Autodesk Inventor part; units mm, degrees
ref_plane "YZ Plane" through (0, 0, 0) normal (1, 0, 0) x (0, 1, 0)
ref_plane "XZ Plane" through (0, 0, 0) normal (0, 1, 0) x (-1, 0, 0)
ref_plane "XY Plane" through (0, 0, 0) normal (0, 0, 1) x (1, 0, 0)
sketch "Sketch1" plane through (0, 0, 0) normal (0, 1, 0) x (-1, 0, 0)
  line L0 (8, 8) -> (-8, 8) construction
  line L1 (-8, 8) -> (-8, -8) construction
  line L2 (-8, -8) -> (8, -8) construction
  line L3 (8, -8) -> (8, 8) construction
  line L4 (8, 8) -> (-8, -8) construction
  line L5 (-8, 8) -> (8, -8) construction
  line L6 (-8.25, 8.25) -> (8.25, 8.25)
  line L7 (8.25, 8.25) -> (8.25, -8.25)
  line L8 (8.25, -8.25) -> (-8.25, -8.25)
  line L9 (-8.25, -8.25) -> (-8.25, 8.25)
  line L10 (-8.25, 8.25) -> (8.25, -8.25) construction
  line L11 (8.25, 8.25) -> (-8.25, -8.25) construction
  line L12 (-10.25, 10.25) -> (10.25, 10.25)
  line L13 (10.25, 10.25) -> (10.25, -10.25)
  line L14 (10.25, -10.25) -> (-10.25, -10.25)
  line L15 (-10.25, -10.25) -> (-10.25, 10.25)
  line L16 (-10.25, 10.25) -> (10.25, -10.25) construction
  line L17 (10.25, 10.25) -> (-10.25, -10.25) construction
  circle A0 centre (2.8, -4.25) radius 1.75
  circle A1 centre (-2.8, -4.25) radius 1.75
  line L18 (7.25, -7.25) -> (-7.25, -7.25)
  line L19 (-7.25, -1.25) -> (7.25, -1.25)
  line L20 (7.25, -1.25) -> (7.25, -7.25)
  line L21 (-7.25, -1.25) -> (-7.25, -7.25)
  line L22 (-6.75, 8.25) -> (-6.75, 10.25)
  line L23 (0, 8.25) -> (0, 10.25)
  point P0 (0, 0)
  point P1 (0, -1.25)
  point P2 (7.25, -4.25)
  dimension "d0" = 16
  dimension "d1" = 16.5
  dimension "d2" = 2
  dimension "d3" = 3.5
  dimension "d4" = 5.6
  dimension "d5" = 2.8
  dimension "d6" = 6
  dimension "d7" = 1
  dimension "d8" = 1
  dimension "d15" = 1.5
extrude "Extrusion1" add sketch "Sketch1" along normal blind 1.5 contours L9 L8 L7 L6 L23 L12 L13 L14 L15 L22
extrude "Extrusion2" add sketch "Sketch1" against normal blind 1.5 contours L9 L8 L7 L6 L23 L12 L13 L14 L15 L22 | L6 L7 L8 L9 | L22 L12 L23 L6
sketch "Sketch2" plane through (0, -1.5, 0) normal (0, -1, 0) x (1, 0, 0)
  line L0 (-10.25, -10.25) -> (10.25, -10.25)
  line L1 (10.25, -10.25) -> (10.25, 10.25)
  line L2 (10.25, 10.25) -> (-10.25, 10.25)
  line L3 (-10.25, 10.25) -> (-10.25, -10.25)
  line L4 (-7.25, -1.25) -> (7.25, -1.25)
  line L5 (7.25, -1.25) -> (7.25, -7.25)
  line L6 (7.25, -7.25) -> (-7.25, -7.25)
  line L7 (-7.25, -7.25) -> (-7.25, -1.25)
  circle A0 centre (2.8, -4.25) radius 1.75
  circle A1 centre (-2.8, -4.25) radius 1.75
  point P0 (0, 0)
extrude "Extrusion3" add sketch "Sketch2" along normal blind 3 contours L3 L2 L1 L0 | L4 L5 L6 L7
fillet "Fillet2" radius 2 4 edges at (-10.25, -1.5, 10.25) (-10.25, -1.5, -10.25) (10.25, -1.5, -10.25) (10.25, -1.5, 10.25)
fillet "Fillet3" radius 0.5 18 edges at (-9.6642, 1.5, 9.6642) (-4.125, 1.5, 10.25) (-9.6642, 1.5, -9.6642) (0, 1.5, -10.25) (9.6642, 1.5, -9.6642) (10.25, 1.5, 0) (9.6642, 1.5, 9.6642) (7.5, 1.5, 10.25) (-10.25, 1.5, 0) (0, 0.75, 10.25) (3.375, 0, 10.25) (6.75, 0.75, 10.25) (-8.25, 0.75, 8.25) (-8.25, 0.75, -8.25) (8.25, 0.75, -8.25) (8.25, 0.75, 8.25) (6.75, 0.75, 8.25) (0, 0.75, 8.25)
chamfer "Chamfer1" distance 0.5 angle 45 10 edges at (1.05, -4.5, -4.25) (-4.55, -4.5, -4.25) (0, -4.5, 10.25) (-9.6642, -4.5, 9.6642) (-10.25, -4.5, 0) (-9.6642, -4.5, -9.6642) (0, -4.5, -10.25) (9.6642, -4.5, -9.6642) (10.25, -4.5, 0) (9.6642, -4.5, 9.6642)
sketch "Sketch3" plane through (0, 0, 0) normal (0, 1, 0) x (1, 0, 0)
  line L0 (7.25, 1.25) -> (-7.25, 1.25)
  line L1 (-7.25, 1.25) -> (-7.25, 7.25)
  line L2 (-7.25, 7.25) -> (7.25, 7.25)
  line L3 (7.25, 7.25) -> (7.25, 1.25)
  arc A0 (7.75, -8.25) -> (8.25, -7.75) centre (7.75, -7.75) ccw
  line L4 (8.25, 7.75) -> (8.25, -7.75)
  arc A1 (8.25, 7.75) -> (7.75, 8.25) centre (7.75, 7.75) ccw
  line L5 (-7.75, 8.25) -> (7.75, 8.25)
  arc A2 (-7.75, 8.25) -> (-8.25, 7.75) centre (-7.75, 7.75) ccw
  line L6 (-8.25, -7.75) -> (-8.25, 7.75)
  arc A3 (-8.25, -7.75) -> (-7.75, -8.25) centre (-7.75, -7.75) ccw
  line L7 (-0.5, -8.25) -> (-7.75, -8.25)
  arc A4 (0, -8.75) -> (-0.5, -8.25) centre (-0.5, -8.75) ccw
  line L8 (0, -9.75) -> (0, -8.75)
  line L9 (6.75, -9.75) -> (0, -9.75)
  line L10 (6.75, -8.75) -> (6.75, -9.75)
  arc A5 (7.25, -8.25) -> (6.75, -8.75) centre (7.25, -8.75) ccw
  line L11 (7.75, -8.25) -> (7.25, -8.25)
  line L12 (-7.25, 1.25) -> (7.25, 1.25)
  line L13 (7.25, 1.25) -> (7.25, -7.25)
  line L14 (7.25, -7.25) -> (-7.25, -7.25)
  line L15 (-7.25, -7.25) -> (-7.25, 1.25)
  point P0 (0, 0)
  dimension "d22" = 1
extrude "Extrusion4" cut sketch "Sketch3" against normal blind 1 contours L13 L14 L15 L0
chamfer "Chamfer2" distance 0.5 angle 45 1 edges at (0, -1, -1.25)
fillet "Fillet4" radius 1 2 edges at (-7.25, -0.5, 7.25) (7.25, -0.5, 7.25)
equation "\"d8\" = d7"
properties part number "Light Pipe Mount - Top"
Build history of the part. All positions in model axes, mm. A direction names the side the tool comes from. Give positions to 0.01 mm unless a question says otherwise; leave off trailing zeros. Order: outer loops, then holes, each group sorted by start corner. A loop starts at its lowest first (then second) coordinate and runs counter-clockwise, first axis right, second up. Notation, with made-up numbers: M 1,65 L 59,65 A10 cw 59,82 Z; hole C 77,71 d10. An arc over 180 degrees is marked long. Return JSON: item names as keys, results as strings.
Q1. Band-saw the part on A-A (y = -3.5). Give the cut face in (x, z), then the cut area to 3 significant figures.
Answer list:
{"outline": "M -10.25,-8.25 A2 ccw -8.25,-10.25 L 8.25,-10.25 A2 ccw 10.25,-8.25 L 10.25,8.25 A2 ccw 8.25,10.25 L -8.25,10.25 A2 ccw -10.25,8.25 Z; hole C -2.8,-4.25 d3.5; hole C 2.8,-4.25 d3.5", "area": "398 mm^2"}
Q2. Band-saw the part on B-B (z = -4.25). Give the cut face in (x, y).
Answer list:
{"outline": "M -10.25,-4 L -9.75,-4.5 L -5.05,-4.5 L -4.55,-4 L -4.55,-1.5 L -7.25,-1.5 L -7.25,0 L -8.25,0 L -8.25,1.5 L -9.75,1.5 A0.5 ccw -10.25,1 Z; M -1.05,-4 L -0.55,-4.5 L 0.55,-4.5 L 1.05,-4 L 1.05,-1.5 L -1.05,-1.5 Z; M 4.55,-4 L 5.05,-4.5 L 9.75,-4.5 L 10.25,-4 L 10.25,1 A0.5 ccw 9.75,1.5 L 8.25,1.5 L 8.25,0 L 7.25,0 L 7.25,-1.5 L 4.55,-1.5 Z"}
Q3. Two-plate mould, pull along Z, no slides. Class faces 1 (the face through (6.75, 1, 9)), 2 (the face through (0, -2, 10.25)), 3 (the face through (-4, 1, 8.25)): pulls with the +Z half, pulls with the -Z half, needs draft (parallel to the pull), parting line crosses it, or undercut.
Answer list:
{"face 1": "needs draft", "face 2": "pulls with the +Z half", "face 3": "undercut"}
Q4. Wall check: probe 1 along Z at (x, y) = (2.8, -2); probe 2 along X at (y, z) = (-0.5, 5.5); probe 3 along X at (y, z) = (0.75, 4). Give the ranges that are in metal, low to high. Write a range as from..to.
Answer list:
{"probe 1": "z = -10.25..-6, -2.5..10.25", "probe 2": "x = -10.25..-7.25, 7.25..10.25", "probe 3": "x = -10.25..-8.25, 8.25..10.25"}
Q5. 3-axis set-ups, long thin cutter, end or side, ignore diameter. For faces 4 (the face through (6.965, -0.507, 6.949)), 5 (the face through (2.42, -2.73, -2.54)), 6 (the face through (0, 1, 9)): which of +Z, -Z, +X, -X, +Y, -Y reach the whole face in a straight line?
Answer list:
{"face 4": "+Y", "face 5": "+Y, -Y", "face 6": "+Z, +Y"}
Q6. Band-saw the part on D-D (y = -1.25). Give the cut face in (x, z).
Answer list:
{"outline": "M -10.25,-8.25 A2 ccw -8.25,-10.25 L 8.25,-10.25 A2 ccw 10.25,-8.25 L 10.25,8.25 A2 ccw 8.25,10.25 L -8.25,10.25 A2 ccw -10.25,8.25 Z; hole M -7.25,-7.25 L 7.25,-7.25 L 7.25,-1 L -7.25,-1 Z"}
Q7. Flat gauge pins, fed straight in: pin 1 (3 mm diameter, centred on x = -5, z = -6, fed in from +Y); pin 2 (4 mm diameter, centred on x = 2, z = 1.5, fed in from +Y); pin 3 (4 mm diameter, centred on x = 2.8, z = -4.25, fed in from +Y). Where does each tip first touch, or does it go through?
Answer list:
{"pin 1": "stops at y = 0", "pin 2": "stops at y = -1", "pin 3": "stops at y = -1.5"}
